from build123d import *

# Parameters (mm, degrees)
EXTRUDE_1_DEPTH = 0.75
SKETCH_2_W      = 6.4
SKETCH_2_H      = 0.5
EXTRUDE_2_DEPTH = 0.15


with BuildPart() as part:
    # 草图1 → 凸台-拉伸1 (new body)
    with BuildSketch(Plane(origin=(0, 0, 0), x_dir=(1, 0, 0), z_dir=(0, 1, 0))):
        Polygon((-1.42, 2.4), (1.42, 2.4), (2.4, 1.42), (2.4, -1.42), (1.42, -2.4), (-1.42, -2.4), (-2.4, -1.42), (-2.4, 1.42), align=None)
    extrude(amount=EXTRUDE_1_DEPTH)

    # 草图2 → 凸台-拉伸2 (add)
    with BuildSketch(Plane.XZ):
        with Locations((0, 1.85)):
            Rectangle(SKETCH_2_W, SKETCH_2_H)
        with Locations((0, -1.85)):
            Rectangle(SKETCH_2_W, SKETCH_2_H)
    extrude(amount=-EXTRUDE_2_DEPTH)


solid = part.part
Read the model definition and answer for the solid it produces. Units are mm, in the model's axes. Round coordinates to 2 decimals unless told otherwise and drop trailing zeros. Order: outer loops, then holes, each group sorted by start corner. A loop starts at its lowest first (then second) coordinate and runs counter-clockwise, first axis right, second up. Notation, with made-up numbers: (3.5, -13) - (12.5, -13) arc R14 ccw to (12.5, 10) - close; hole circle Ø7 at (83, -16). An arc over 180 degrees is marked (long way). Use one line per item in the form item = value. Start each with the question number.
(1) The part is cut by section B-B (y = 0.3). Give the vertices of the cut face in (x, z), then the cut area to 3 significant figures.
(2) The part is cut by section C-C (z = 2). Give the vertices of the cut face in (x, y), then the cut area to 3 significant figures.
(3) A flat-ended cylindrical pin translates along its axis: pin 1 Ø0.6 at (x, z) = (-2.5, 2) entering from +Y. Find the tip coordinate at first contact, or state that the pin passes through.
(4) The part is cut by section A-A (x = 2.5). Give the vertices of the cut face in (y, z), then the cut area to 3 significant figures.
(5) The part is cut by section D-D (x = 1.5). Give the vertices of the cut face in (y, z).
(6) Find the intervals of material crossed by line 1 along Z through (x, y) = (2.75, 0.1); line 2 along X through (y, z) = (0.2, -1); line 3 along Z through (x, y) = (-2, 0.2), in increasing order. Write a range as from..to.
Checked values:
q1.outline = (-2.4, -1.42) - (-1.42, -2.4) - (1.42, -2.4) - (2.4, -1.42) - (2.4, 1.42) - (1.42, 2.4) - (-1.42, 2.4) - (-2.4, 1.42) - close
q1.area = 21.1 mm^2
q2.outline = (-3.2, 0) - (3.2, 0) - (3.2, 0.15) - (1.82, 0.15) - (1.82, 0.75) - (-1.82, 0.75) - (-1.82, 0.15) - (-3.2, 0.15) - close
q2.area = 3.14 mm^2
q3.pin_1 = 0.15
q4.outline = (0, -2.1) - (0.15, -2.1) - (0.15, -1.6) - (0, -1.6) - close; (0, 1.6) - (0.15, 1.6) - (0.15, 2.1) - (0, 2.1) - close
q4.area = 0.150 mm^2
q5.outline = (0, -2.32) - (0.75, -2.32) - (0.75, 2.32) - (0, 2.32) - close
q6.line_1 = -2.1..-1.6, 1.6..2.1
q6.line_2 = -2.4..2.4
q6.line_3 = -1.82..1.82
